```python
from build123d import *

# Parameters (mm, degrees)
SKETCH2_R           = 5
BOSS_EXTRUDE1_DEPTH = 10
FILLET1_R           = 2


with BuildPart() as part:
    # Sketch2 → Boss-Extrude1 (new body)
    with BuildSketch(Plane.XY):
        with BuildLine():
            ThreePointArc((-136.248221627, 62.740912517), (-147.363336048, 28.000842642), (-149.764900792, -8.394908626))
            ThreePointArc((-149.764900792, -8.394908626), (-132.116158495, -15.482544811), (-137.975293762, 2.611189609))
            ThreePointArc((-137.975293762, 2.611189609), (-135.574269165, 25.760775231), (-129.317107469, 48.177647472))
            ThreePointArc((-129.317107469, 48.177647472), (-117.229857172, 62.861348354), (-136.248221627, 62.740912517))
        make_face()
        with Locations((-126.710846113, 58.349048641)):
            Circle(SKETCH2_R, mode=Mode.SUBTRACT)
        with Locations((-139.281357736, -7.807265022)):
            Circle(SKETCH2_R, mode=Mode.SUBTRACT)
    extrude(amount=BOSS_EXTRUDE1_DEPTH)

    # Fillet1
    fillet1_edges = [part.edges().sort_by_distance(p)[0] for p in [
        (-147.363336048, 28.000842642, 10),
        (-132.116158495, -15.482544811, 10),
        (-135.574269165, 25.760775231, 10),
        (-132.116158495, -15.482544811, 0),
        (-147.363336048, 28.000842642, 0),
        (-117.229857172, 62.861348354, 0),
        (-135.574269165, 25.760775231, 0),
        (-117.229857172, 62.861348354, 10),
        (-137.975293762, 2.611189609, 5),
        (-129.317107469, 48.177647472, 5),
    ]]
    fillet(fillet1_edges, radius=FILLET1_R)


solid = part.part
```
CAD build for the part. Positions are in the model's coordinates, mm. A direction names the side the tool comes from. Give positions to 0.01 mm unless a question says otherwise; leave off trailing zeros. Put each result on its own line as item: value. Start each with the question number.
(1) Drill centre lines: line 1 along Y through (x, z) = (-124.5, 6); line 2 along X through (y, z) = (-12, 5.5); line 3 along Y through (x, z) = (-139, 8). Where is each one in solid material? Low to high.
(2) Which spindle directions (+Z, -Z, +X, -X, +Y, -Y) get a long thin tool onto all of the face, cutting with end or side? Do faces 1 (the cylindrical face through (-135.63, 25.46, 4.96)), 2 (the cylindrical face through (-132.951, -16.184, 4.958)). Say none if no direction does.
(3) Saw through at A-A, the plane z = 6. Give the number of separate pieces and of enclosed holes in the cut face, then the cut area to 3 significant figures.
(4) Flat gauge pins, fed straight in: pin 1 Ø8 at (x, y) = (-131.5, 29.5) entering from +Z; pin 2 Ø6 at (x, y) = (-126.71, 58.35) entering from +Z; pin 3 Ø2 at (x, z) = (-134, 2.5) entering from -Y; pin 4 Ø2 at (x, z) = (-136, 2) entering from -Y. Where does each tip first touch, or does it go through?
Check result:
1. line 1: y = 48.08 to 53.86, 62.83 to 68.61
1. line 2: x = -148.91 to -142.01, -136.56 to -129.65
1. line 3: y = -18.3 to -12.8, -2.82 to 56.38
2. face 1: +Z, -Z, +X
2. face 2: +Z, -Z
3. separate pieces: 1
3. enclosed holes: 2
3. area: 1,170 mm2
4. pin 1: stops at z = 9.58
4. pin 2: passes through
4. pin 3: stops at y = -17.39
4. pin 4: stops at y = -18.06
